```python
from build123d import *

# Parameters (mm, degrees)
ESBO_O1_R                = 1.6
ESBO_O1_R_2              = 3
RESSALTO_EXTRUS_O1_DEPTH = 6
FILETE1_R                = 5
FILETE2_R                = 2.6


with BuildPart() as part:
    # Esboço1 → Ressalto-extrusão1 (new body)
    with BuildSketch(Plane.XY):
        with BuildLine():
            Line((-7.5, 26.678233731), (-7.5, -38.58638145))
            Line((-7.5, -38.58638145), (7.5, -38.58638145))
            Line((7.5, -38.58638145), (7.5, 38.58638145))
            Line((7.5, 38.58638145), (-7.5, 38.58638145))
            Line((-7.5, 38.58638145), (-7.5, 33.136612343))
            ThreePointArc((-7.5, 33.136612343), (-4.653230591, 33.430458901), (-1.795586451, 33.58638145))
            ThreePointArc((-1.795586451, 33.58638145), (1.5, 30.484912453), (-1.601468997, 27.189326002))
            ThreePointArc((-1.601468997, 27.189326002), (-4.557903938, 27.016522573), (-7.5, 26.678233731))
        make_face()
        with Locations((0, -33.58638145)):
            Circle(ESBO_O1_R, mode=Mode.SUBTRACT)
        with Locations((0, -25.58638145)):
            Circle(ESBO_O1_R_2, mode=Mode.SUBTRACT)
        with Locations((0, -17.58638145)):
            Circle(ESBO_O1_R, mode=Mode.SUBTRACT)
    extrude(amount=RESSALTO_EXTRUS_O1_DEPTH)

    # Filete1
    filete1_edges = [part.edges().sort_by_distance(p)[0] for p in [
        (7.5, 38.58638145, 3),
        (7.5, -38.58638145, 3),
        (-7.5, -38.58638145, 3),
    ]]
    fillet(filete1_edges, radius=FILETE1_R)

    # Filete2
    filete2_edges = [part.edges().sort_by_distance(p)[0] for p in [
        (-7.5, 38.58638145, 3),
    ]]
    fillet(filete2_edges, radius=FILETE2_R)


solid = part.part
```
CAD build for the part. Positions are in the model's coordinates, mm. A direction names the side the tool comes from. Round coordinates to 2 decimals unless told otherwise and drop trailing zeros. Write each loop counter-clockwise with the first axis right and the second up, starting at its lowest first coordinate (ties: lowest second). Pieces come first, ordered by that corner, then holes.
Item 1: Band-saw the part on C-C on x = 0. Write the cut outline in (y, z), then the cut area to 3 significant figures.
Filled in:
outline: (-38.59, 0) - (-35.19, 0) - (-35.19, 6) - (-38.59, 6) - close; (-31.99, 0) - (-28.59, 0) - (-28.59, 6) - (-31.99, 6) - close; (-22.59, 0) - (-19.19, 0) - (-19.19, 6) - (-22.59, 6) - close; (-15.99, 0) - (27.68, 0) - (27.68, 6) - (-15.99, 6) - close; (33.1, 0) - (38.59, 0) - (38.59, 6) - (33.1, 6) - close
area: 356 mm2
Item 2: Mould opens along Y. For faces 1 (the cylindrical face through (5.996, -37.161, 3.042)), 2 (the flat face through (0, 1, 0)), 3 (the cylindrical face through (-1.27, -18.56, 2.96)) say: released by +Y, released by -Y, zero draft, split by the parting line, or undercut.
Filled in:
face 1: released by -Y
face 2: zero draft
face 3: undercut
Item 3: Drop a flat-ended pin along its axis: pin 1 Ø1.5 at (x, z) = (3.5, 2) entering from -Y. Give the stop position or say it passes through.
Filled in:
pin 1: stops at y = -38.58
Item 4: Tool access for faces 4 (the cylindrical face through (-4.693, 33.427, 2.958)), 5 (the cylindrical face through (-4.52, 27.02, 2.96)), 6 (the flat face through (-7.5, 35, 3)): list every direction of +Z, -Z, +X, -X, +Y, -Y with a clear straight run to the whole face (end or side of a thin tool).
Filled in:
face 4: +Z, -Z
face 5: +Z, -Z, -X
face 6: +Z, -Z, -X, +Y, -Y
Item 5: Band-saw the part on B-B on z = 1.4. Write the cut outline in (x, y), then the cut area to 3 significant figures.
Filled in:
outline: (-7.5, -33.59) arc R5 ccw to (-2.5, -38.59) - (2.5, -38.59) arc R5 ccw to (7.5, -33.59) - (7.5, 33.59) arc R5 ccw to (2.5, 38.59) - (-4.9, 38.59) arc R2.6 ccw to (-7.5, 35.99) - (-7.5, 33.14) arc R59.2 cw to (-1.8, 33.59) arc R3.2 cw to (-1.6, 27.19) arc R52.8 ccw to (-7.5, 26.68) - close; hole circle Ø6 at (0, -25.59); hole circle Ø3.2 at (0, -33.59); hole circle Ø3.2 at (0, -17.59)
area: 1,040 mm2
Item 6: Band-saw the part on D-D on x = 6. Write the cut outline in (y, z), then the cut area to 3 significant figures.
Filled in:
outline: (-37.16, 0) - (37.16, 0) - (37.16, 6) - (-37.16, 6) - close
area: 446 mm2
Item 7: Band-saw the part on A-A on y = -23.5. Write the cut outline in (x, z).
Filled in:
outline: (-7.5, 0) - (-2.16, 0) - (-2.16, 6) - (-7.5, 6) - close; (2.16, 0) - (7.5, 0) - (7.5, 6) - (2.16, 6) - close
Item 8: Drill centre lines: L1, parallel to Y at x = 1.25, z = 0.6; L2, parallel to Y at x = -2, z = 2.85; L3, parallel to Y at x = 0, z = 3.6. Where is each one in solid material? Low to high.
Filled in:
L1: y = -38.59 to -34.59, -32.59 to -28.31, -22.86 to -18.59, -16.59 to 29.14, 31.63 to 38.59
L2: y = -38.59 to -27.82, -23.35 to 27.18, 33.58 to 38.59
L3: y = -38.59 to -35.19, -31.99 to -28.59, -22.59 to -19.19, -15.99 to 27.68, 33.1 to 38.59
